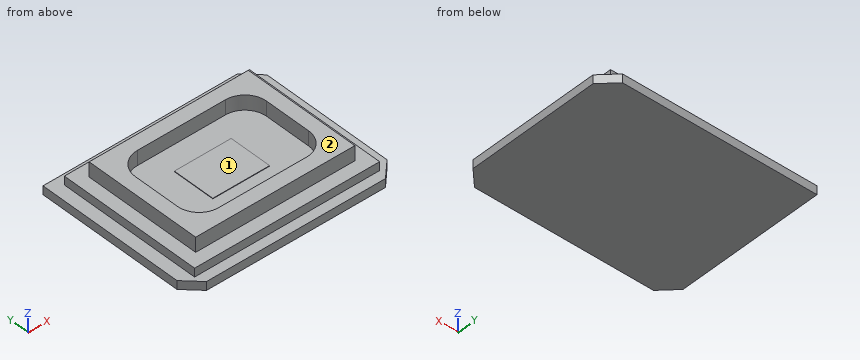
Autodesk Inventor part; units mm, degrees
ref_plane "YZ Plane" through (0, 0, 0) normal (1, 0, 0) x (0, 1, 0)
ref_plane "XZ Plane" through (0, 0, 0) normal (0, 1, 0) x (-1, 0, 0)
ref_plane "XY Plane" through (0, 0, 0) normal (0, 0, 1) x (1, 0, 0)
sketch "Sketch1" plane through (0, 0, 0) normal (0, 0, 1) x (1, 0, 0)
  line L0 (3, 0) -> (40.64, 0)
  line L1 (37.64, 31.75) -> (0, 31.75)
  line L2 (0, 31.75) -> (0, 3)
  line L3 (37.64, 31.75) -> (40.64, 28.75)
  line L4 (3, 0) -> (0, 3)
  line L5 (40.64, 3) -> (37.64, 0)
  line L6 (40.64, 28.75) -> (40.64, 3)
  point P0 (0, 0)
  dimension "d4" = 3
  dimension "d5" = 45
  dimension "d6" = 45
  dimension "d7" = 3
  dimension "d8" = 31.75
  dimension "d9" = 40.64
  dimension "d10" = 3
extrude "Extrusion1" add sketch "Sketch1" along normal blind 1.651
sketch "Sketch2" plane through (0, 0, 1.651) normal (0, 0, 1) x (1, 0, 0)
  line L0 (2.413, 29.845) -> (38.227, 29.845)
  line L1 (38.227, 29.845) -> (38.227, 1.905)
  line L2 (38.227, 1.905) -> (2.413, 1.905)
  line L3 (2.413, 1.905) -> (2.413, 29.845)
  line L4 (0, 31.75) -> (0, 3)
  line L5 (3, 0) -> (37.64, 0)
  line L6 (40.64, 3) -> (40.64, 28.75)
  point P0 (0, 0)
  point P1 (0, 17.375)
  point P2 (20.32, 1.905)
  point P3 (20.32, 0)
  point P4 (38.227, 15.875)
  point P5 (40.64, 15.875)
  dimension "d13" = 27.94
  dimension "d14" = 35.814
extrude "Extrusion2" add sketch "Sketch2" along normal blind 1.65
sketch "Sketch3" plane through (0, 0, 3.301) normal (0, 0, 1) x (1, 0, 0)
  line L0 (4.92, 27.305) -> (35.72, 27.305)
  line L1 (35.72, 27.305) -> (35.72, 4.445)
  line L2 (35.72, 4.445) -> (4.92, 4.445)
  line L3 (4.92, 4.445) -> (4.92, 27.305)
  line L4 (2.413, 29.845) -> (2.413, 1.905)
  line L5 (3, 0) -> (37.64, 0)
  point P0 (0, 0)
  point P1 (4.92, 15.875)
  point P2 (2.413, 15.875)
  point P3 (20.32, 4.445)
  point P4 (20.32, 0)
  dimension "d17" = 22.86
  dimension "d18" = 30.8
extrude "Extrusion3" add sketch "Sketch3" along normal blind 2.83
sketch "Sketch4" plane through (0, 0, 6.131) normal (0, 0, 1) x (1, 0, 0)
  line L0 (11.82, 24.575) -> (28.82, 24.575)
  line L1 (33.02, 20.375) -> (33.02, 11.375)
  line L2 (28.82, 7.175) -> (11.82, 7.175)
  line L3 (7.62, 11.375) -> (7.62, 20.375)
  line L4 (4.92, 27.305) -> (4.92, 4.445)
  line L5 (2.413, 1.905) -> (38.227, 1.905)
  arc A0 (7.62, 11.375) -> (11.82, 7.175) centre (11.82, 11.375) ccw
  arc A1 (11.82, 24.575) -> (7.62, 20.375) centre (11.82, 20.375) ccw
  arc A2 (33.02, 20.375) -> (28.82, 24.575) centre (28.82, 20.375) ccw
  arc A3 (28.82, 7.175) -> (33.02, 11.375) centre (28.82, 11.375) ccw
  point P0 (0, 0)
  point P1 (7.62, 24.575)
  point P2 (33.02, 7.175)
  point P3 (7.62, 7.175)
  point P4 (7.62, 15.875)
  point P5 (4.92, 15.875)
  point P6 (20.32, 7.175)
  point P7 (20.32, 1.905)
  dimension "d21" = 17.4
  dimension "d22" = 25.4
  dimension "d23" = 4.2
extrude "Extrusion4" cut sketch "Sketch4" against normal blind 2.83
sketch "Sketch5" plane through (0, 0, 3.301) normal (0, 0, 1) x (1, 0, 0)
  line L0 (25.82, 11.75) -> (14.82, 11.75)
  line L1 (14.82, 11.75) -> (14.82, 20)
  line L2 (14.82, 20) -> (25.82, 20)
  line L3 (25.82, 20) -> (25.82, 11.75)
  line L4 (7.62, 11.375) -> (7.62, 20.375)
  line L5 (28.82, 7.175) -> (11.82, 7.175)
  point P0 (0, 0)
  point P1 (14.82, 15.875)
  point P2 (7.62, 15.875)
  point P3 (20.32, 11.75)
  point P4 (20.32, 7.175)
  dimension "d26" = 11
  dimension "d27" = 8.25
extrude "Extrusion5" add sketch "Sketch5" along normal blind 0.1
properties part number "DLP"
CAD build for the part. Positions are in the model's coordinates, mm. Face numbers are marked on the shaded views. A direction names the side the tool comes from. Coordinates: 2 decimals unless noted, no trailing zeros. Loops run counter-clockwise (first coordinate to the right, second up) from the corner with the lowest first, then second, coordinate; pieces in that order, holes last. Notation, with made-up numbers: (40, 35.5) - (99, 35.5) arc R26 cw to (99, 73.5) - close; hole circle Ø11 at (40, 42). An arc over 180 degrees is marked (long way). Use CSV: the item, a comma, the result in double quotes. Start each with the question number.
Q1. Cut at D-D, the plane z = 2.75. List the corners of the cut face in (x, y) (3 decimals), then the cut area to 3 significant figures.
Q2. Probe probe 1 along Y at (x, z) = (21, 3.5) (3 decimals); probe 2 along X at (y, z) = (6.5, 1.75); probe 3 along Z at (x, y) = (6.5, 2.5). List the from-to ranges inside material, lowest first. Write a range as from..to.
Q3. 3-axis set-ups, long thin cutter, end or side, ignore diameter. For the marked faces 1 and 2: which of +Z, -Z, +X, -X, +Y, -Y reach the whole face in a straight line?
Q4. Cut at B-B, the plane x = 16. List the corners of the cut face in (y, z) (3 decimals), then the cut area to 3 significant figures.
Q5. Cut at C-C, the plane y = 13.5. List the corners of the cut face in (x, z).
Q6. Cut at A-A, the plane z = 5. List the corners of the cut face in (x, y) (3 decimals), then the cut area to 3 significant figures.
Q7. Drop flat-ended pins along their axis: P1, Ø1.5, axis at y = 11, z = 5, coming from the +X side; P2, Ø9, axis at x = 23, y = 14.5, coming from the +Z side; P3, Ø3, axis at y = 16, z = 4, coming from the -X side; P4, Ø1.8, axis at x = 25.5, z = 2, coming from the +Y side. Give the stop position or say it passes through.
Here are the results:
1,outline,"(2.413, 1.905) - (38.227, 1.905) - (38.227, 29.845) - (2.413, 29.845) - close"
1,area,"1,000 mm2"
2,probe 1,"4.445..7.175, 24.575..27.305"
2,probe 2,"2.41..38.23"
2,probe 3,"0..3.3"
3,face 1,"+Z"
3,face 2,"+Z, +X, -X, +Y, -Y"
4,outline,"(0, 0) - (31.75, 0) - (31.75, 1.651) - (29.845, 1.651) - (29.845, 3.301) - (27.305, 3.301) - (27.305, 6.131) - (24.575, 6.131) - (24.575, 3.301) - (20, 3.301) - (20, 3.401) - (11.75, 3.401) - (11.75, 3.301) - (7.175, 3.301) - (7.175, 6.131) - (4.445, 6.131) - (4.445, 3.301) - (1.905, 3.301) - (1.905, 1.651) - (0, 1.651) - close"
4,area,"115 mm2"
5,outline,"(0, 0) - (40.64, 0) - (40.64, 1.65) - (38.23, 1.65) - (38.23, 3.3) - (35.72, 3.3) - (35.72, 6.13) - (33.02, 6.13) - (33.02, 3.3) - (25.82, 3.3) - (25.82, 3.4) - (14.82, 3.4) - (14.82, 3.3) - (7.62, 3.3) - (7.62, 6.13) - (4.92, 6.13) - (4.92, 3.3) - (2.41, 3.3) - (2.41, 1.65) - (0, 1.65) - close"
6,outline,"(4.92, 4.445) - (35.72, 4.445) - (35.72, 27.305) - (4.92, 27.305) - close; hole (7.62, 11.375) arc R4.2 ccw to (11.82, 7.175) - (28.82, 7.175) arc R4.2 ccw to (33.02, 11.375) - (33.02, 20.375) arc R4.2 ccw to (28.82, 24.575) - (11.82, 24.575) arc R4.2 ccw to (7.62, 20.375) - close"
6,area,"277 mm2"
7,P1,"x = 35.72"
7,P2,"z = 3.4"
7,P3,"x = 2.41"
7,P4,"y = 31.75"
